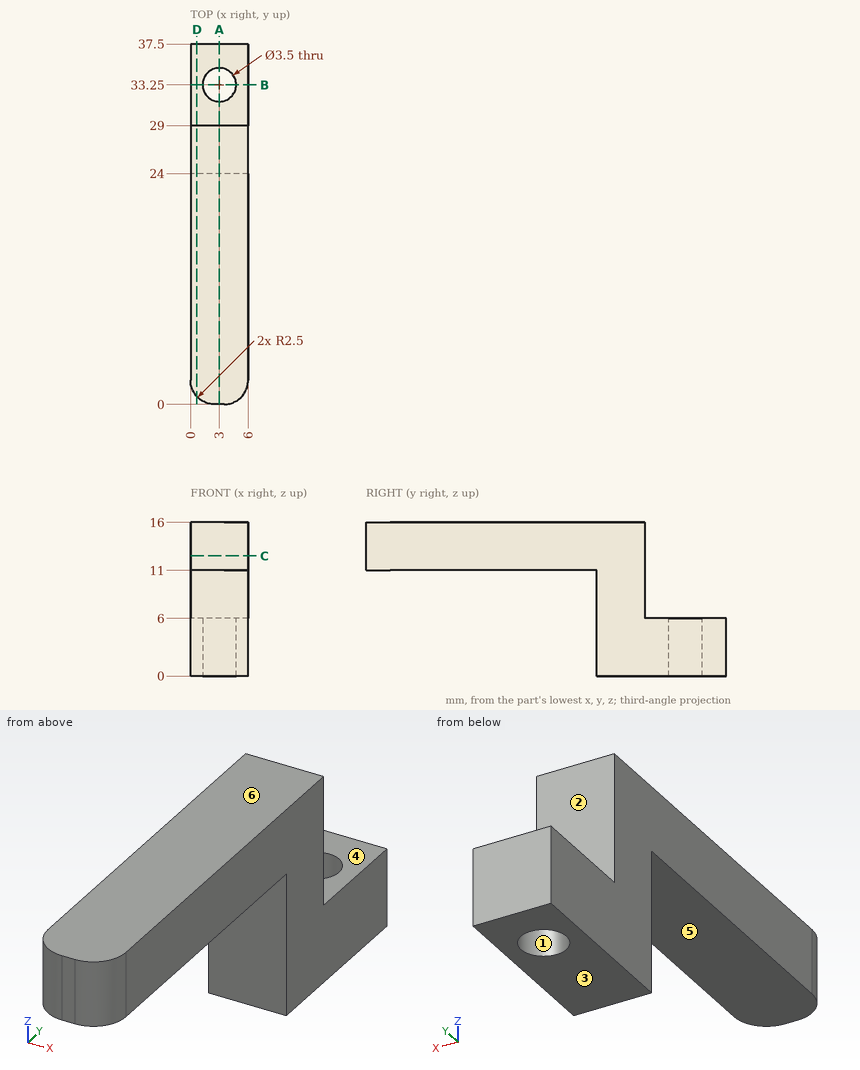
Can you work these out from the drawing? Everything is in mm from the part's minimum corner. A direction names the side the tool comes from. Give positions to 0.01 mm unless a question says otherwise; leave off trailing zeros. Loops run counter-clockwise (first coordinate to the right, second up) from the corner with the lowest first, then second, coordinate; pieces in that order, holes last. Notation, with made-up numbers: (-1.5, 22) -> (57.5, 22) arc R16 ccw to (57.5, 36) -> close; hole circle Ø11 at (-15.75, 4.5). An arc over 180 degrees is marked (long way). Return JSON: item names as keys, results as strings.
Q1. On a 3-axis mill with a long thin cutter (end or side, diameter ignored), from which of +Z, -Z, +X, -X, +Y, -Y can I reach the whole of each face in a straight line? I mean the marked faces 4, 5 and 6. Say none if no direction works.
Checks:
{"face 4": "+Z, +X, -X, +Y", "face 5": "-Z, +X, -X, -Y", "face 6": "+Z, +X, -X, +Y, -Y"}
Q2. I want a section at C-C, the plane z = 12.5. List the corners of the cut face in (x, y) for me.
Checks:
{"outline": "(0, 2.5) arc R2.5 ccw to (2.5, 0) -> (3.5, 0) arc R2.5 ccw to (6, 2.5) -> (6, 29) -> (0, 29) -> close"}
Q3. I want a section at A-A, the plane x = 3. List the corners of the cut face in (y, z) for me.
Checks:
{"outline": "(0, 11) -> (24, 11) -> (24, 0) -> (31.5, 0) -> (31.5, 6) -> (29, 6) -> (29, 16) -> (0, 16) -> close; (35, 0) -> (37.5, 0) -> (37.5, 6) -> (35, 6) -> close"}
Q4. For pin 1 Ø1.8 at (x, y) = (3.5, 8.5) entering from -Z; pin 2 Ø1.8 at (x, z) = (2, 3.5) entering from -Y; pin 3 Ø3 at (x, z) = (1, 8) entering from +Y, each with a flat end and sliding along its axis, tell me the tip position at first contact or that it passes through.
Checks:
{"pin 1": "stops at z = 11", "pin 2": "stops at y = 24", "pin 3": "stops at y = 29"}
Q5. I want a section at B-B, the plane y = 33.25. List the corners of the cut face in (x, z) for me, then the cut area to 3 significant figures.
Checks:
{"outline": "(0, 0) -> (1.25, 0) -> (1.25, 6) -> (0, 6) -> close; (4.75, 0) -> (6, 0) -> (6, 6) -> (4.75, 6) -> close", "area": "15.0 mm2"}
Q6. I need wall thicknesses on probe 1 along X at (y, z) = (33.25, 2.05); probe 2 along Y at (x, z) = (3, 1.85); probe 3 along Z at (x, y) = (4.35, 15.5). Which ranges of each line are inside material? Lowest first, please.
Checks:
{"probe 1": "x = 0 to 1.25, 4.75 to 6", "probe 2": "y = 24 to 31.5, 35 to 37.5", "probe 3": "z = 11 to 16"}
Q7. We'd pull the mould along Y, two halves only. Please class the marked faces 1, 2 and 3: released by +Y, released by -Y, zero draft, split by the parting line, or undercut.
Checks:
{"face 1": "undercut", "face 2": "released by +Y", "face 3": "zero draft"}
Q8. I want a section at D-D, the plane x = 0.65. List the corners of the cut face in (y, z) for me.
Checks:
{"outline": "(0.82, 11) -> (24, 11) -> (24, 0) -> (37.5, 0) -> (37.5, 6) -> (29, 6) -> (29, 16) -> (0.82, 16) -> close"}
